from build123d import *

# Parameters (mm, degrees)
F1_DEPTH = 250


with BuildPart() as f1:
    # F0 (on Front) → F1 (new body, symmetric)
    with BuildSketch(Plane.XZ):
        with BuildLine():
            ThreePointArc((50, 30), (44.1421356237, 44.1421356237), (30, 50))
            Line((30, 50), (-30, 50))
            ThreePointArc((-30, 50), (-44.1421356237, 44.1421356237), (-50, 30))
            Line((-50, 30), (-50, -30))
            ThreePointArc((-50, -30), (-44.1421356237, -44.1421356237), (-30, -50))
            Line((-30, -50), (30, -50))
            ThreePointArc((30, -50), (44.1421356237, -44.1421356237), (50, -30))
            Line((50, -30), (50, 30))
        make_face()
        with BuildLine():
            Line((-40, -30), (-40, 30))
            ThreePointArc((-40, 30), (-37.0710678119, 37.0710678119), (-30, 40))
            Line((-30, 40), (30, 40))
            ThreePointArc((30, 40), (37.0710678119, 37.0710678119), (40, 30))
            Line((40, 30), (40, -30))
            ThreePointArc((40, -30), (37.0710678119, -37.0710678119), (30, -40))
            Line((30, -40), (-30, -40))
            ThreePointArc((-30, -40), (-37.0710678119, -37.0710678119), (-40, -30))
        make_face(mode=Mode.SUBTRACT)
    extrude(amount=F1_DEPTH, both=True)


solid = f1.part
Geometry: final body of the model. Coordinates: model frame, mm. A direction names the side the tool comes from. Coordinates: 2 decimals unless noted, no trailing zeros. Order: outer loops, then holes, each group sorted by start corner. A loop starts at its lowest first (then second) coordinate and runs counter-clockwise, first axis right, second up. Notation, with made-up numbers: (65, -1) - (119, -1) arc R16 cw to (119, 18) - close; hole circle Ø3 at (-7, 61.5). An arc over 180 degrees is marked (long way). Use one line per item in the form item = value.
1) Section A-A (x = 13). Return loops of the section in (y, z).
Solutions:
outline = (-250, -50) - (250, -50) - (250, -40) - (-250, -40) - close; (-250, 40) - (250, 40) - (250, 50) - (-250, 50) - close
2) Pin query (flat end, axial travel): pin 1 (3 mm diameter, centred on y = -1, z = -34, fed in from -X); pin 2 (2 mm diameter, centred on x = -37.5, y = -192, fed in from +Z). Return the tip coordinate at first contact, or that it passes through.
Solutions:
pin_1 = -49.84
pin_2 = 48.91
3) Set-up query: faces 1 (the face through (-43.986, -3.5, 44.297)), 2 (the face through (37.15, -3.5, -36.99)). Return all of +Z, -Z, +X, -X, +Y, -Y with unobstructed straight access to the full face (end or side cutting, diameter ignored); none if empty.
Solutions:
face_1 = +Z, -X, +Y, -Y
face_2 = +Y, -Y
4) Ray query, L1, parallel to X at y = 84, z = -16; L2, parallel to X at y = 228.5, z = -38. Return the intervals inside material, ascending.
Solutions:
L1 = -50 to -40, 40 to 50
L2 = -48.33 to -36, 36 to 48.33
5) Mould query, pull axis X, two halves, no side actions, for faces 3 (the face through (36.99, -3.5, 37.15)), 4 (the face through (-41, 250, 0)), 5 (the face through (43.986, -3.5, -44.297)). Classes: +X half, -X half, draft (parallel to the pull), parting line (faces both ways), or undercut.
Solutions:
face_3 = undercut
face_4 = draft
face_5 = +X half
6) Section B-B (y = 50). Return loops of the section in (x, z).
Solutions:
outline = (-50, -30) arc R20 ccw to (-30, -50) - (30, -50) arc R20 ccw to (50, -30) - (50, 30) arc R20 ccw to (30, 50) - (-30, 50) arc R20 ccw to (-50, 30) - close; hole (-40, -30) arc R10 ccw to (-30, -40) - (30, -40) arc R10 ccw to (40, -30) - (40, 30) arc R10 ccw to (30, 40) - (-30, 40) arc R10 ccw to (-40, 30) - close
7) Section C-C (z = 20). Return loops of the section in (x, y), then the cut area to 3 significant figures.
Solutions:
outline = (-50, -250) - (-40, -250) - (-40, 250) - (-50, 250) - close; (40, -250) - (50, -250) - (50, 250) - (40, 250) - close
area = 10,000 mm^2
